Autodesk Inventor part; units mm, degrees
ref_plane "YZ Plane" through (0, 0, 0) normal (1, 0, 0) x (0, 1, 0)
ref_plane "XZ Plane" through (0, 0, 0) normal (0, 1, 0) x (-1, 0, 0)
ref_plane "XY Plane" through (0, 0, 0) normal (0, 0, 1) x (1, 0, 0)
sketch "Sketch1" plane through (0, 0, 0) normal (0, 0, 1) x (1, 0, 0)
  line L0 (0, 0) -> (15, 0)
  line L1 (15, 0) -> (15, 10)
  line L2 (15, 10) -> (0, 10)
  line L3 (0, 10) -> (0, 0)
  line L4 (1, 9) -> (14, 9)
  line L5 (14, 9) -> (14, 1)
  line L6 (14, 1) -> (1, 1)
  line L7 (1, 1) -> (1, 9)
  dimension "d0" = 15
  dimension "d1" = 10
  dimension "d2" = 13
  dimension "d3" = 8
  dimension "d4" = 1
  dimension "d5" = 1
extrude "Extrusion1" add sketch "Sketch1" along normal blind 28
sketch "Sketch2" plane through (0, 10, 0) normal (0, 1, 0) x (1, 0, 0)
  line L0 (15, 0) -> (0, 0)
  line L1 (0, 0) -> (0, -28)
  line L2 (15, -28) -> (0, -28)
  line L3 (15, 0) -> (15, -28)
  circle A0 centre (7.5, -5) radius 1.5
  circle A1 centre (7.5, -18) radius 1.5
  dimension "d8" = 3
  dimension "d9" = 3
  dimension "d10" = 7.5
  dimension "d11" = 7.5
  dimension "d12" = 5
  dimension "d13" = 10
extrude "Extrusion2" cut sketch "Sketch2" against normal up to surface (10 mm away) contours A0 | A1
sketch "Sketch3" plane through (15, 0, 0) normal (1, 0, 0) x (0, 0, -1)
  line L0 (0, 0) -> (0, 10)
  line L1 (0, 10) -> (-28, 10)
  line L2 (-28, 0) -> (-28, 10)
  line L3 (0, 0) -> (-28, 0)
  circle A0 centre (-9, 5) radius 1.5
  circle A1 centre (-23, 5) radius 1.5
  dimension "d16" = 3
  dimension "d17" = 5
  dimension "d18" = 9
  dimension "d21" = 3
  dimension "d22" = 5
  dimension "d23" = 5
extrude "Extrusion3" cut sketch "Sketch3" against normal up to surface (15 mm away) contours A0 | A1
properties part number "profile3" material "Aluminum 6061, Welded"
Source: CAD feature listing. Evaluate the final solid. Frame: model axes, mm. A direction names the side the tool comes from. Round coordinates to 2 decimals unless told otherwise and drop trailing zeros. Order: outer loops, then holes, each group sorted by start corner. A loop starts at its lowest first (then second) coordinate and runs counter-clockwise, first axis right, second up. Notation, with made-up numbers: (49, 60.5) -> (68, 60.5) arc R21 ccw to (68, 76.5) -> close; hole circle Ø6 at (51.25, -23.5). An arc over 180 degrees is marked (long way). Answer as CSV lines item,"result".
Item 1: Section B-B, the plane x = 7.5. Return loops of the section in (y, z).
A:
outline,"(0, 0) -> (1, 0) -> (1, 3.5) -> (0, 3.5) -> close; (0, 6.5) -> (1, 6.5) -> (1, 16.5) -> (0, 16.5) -> close; (0, 19.5) -> (1, 19.5) -> (1, 28) -> (0, 28) -> close; (9, 0) -> (10, 0) -> (10, 3.5) -> (9, 3.5) -> close; (9, 6.5) -> (10, 6.5) -> (10, 16.5) -> (9, 16.5) -> close; (9, 19.5) -> (10, 19.5) -> (10, 28) -> (9, 28) -> close"
Item 2: Section A-A, the plane y = 1.75. Return loops of the section in (x, z), plus the area to 3 significant figures.
A:
outline,"(0, 0) -> (1, 0) -> (1, 28) -> (0, 28) -> close; (14, 0) -> (15, 0) -> (15, 28) -> (14, 28) -> close"
area,"56.0 mm²"
Item 3: Section C-C, the plane z = 5. Return loops of the section in (x, y), plus the area to 3 significant figures.
A:
outline,"(0, 0) -> (6, 0) -> (6, 1) -> (1, 1) -> (1, 9) -> (6, 9) -> (6, 10) -> (0, 10) -> close; (9, 0) -> (15, 0) -> (15, 10) -> (9, 10) -> (9, 9) -> (14, 9) -> (14, 1) -> (9, 1) -> close"
area,"40.0 mm²"
Item 4: Line query: L1, parallel to Z at x = 7.5, y = 9.4; L2, parallel to Y at x = 13, z = 2.5; L3, parallel to Y at x = 0.7, z = 23. Output: solid intervals per line, ascending.
A:
L1,"0 to 3.5, 6.5 to 16.5, 19.5 to 28"
L2,"0 to 1, 9 to 10"
L3,"0 to 3.5, 6.5 to 10"
Item 5: Section D-D, the plane x = 10. Return loops of the section in (y, z), plus the area to 3 significant figures.
A:
outline,"(0, 0) -> (1, 0) -> (1, 28) -> (0, 28) -> close; (9, 0) -> (10, 0) -> (10, 28) -> (9, 28) -> close"
area,"56.0 mm²"
Item 6: Reachability of faces 4 (the face through (7, 0, 14)), 5 (the face through (1, 5, 14)) from +Z, -Z, +X, -X, +Y, -Y: full face, straight path, thin tool, end or side. Return the list, or none.
A:
face 4,"+Z, -Z, +X, -X, -Y"
face 5,"+Z, -Z"
Item 7: Pull-direction query (Z, two-part tool) for faces 1 (the face through (6.39, 9.51, 3.99)), 2 (the face through (7.4, 0.6, 28)), 3 (the face through (8, 10, 14)); classes: pulls with the +Z half, pulls with the -Z half, needs draft (parallel to the pull), parting line crosses it, or undercut.
A:
face 1,"undercut"
face 2,"pulls with the +Z half"
face 3,"needs draft"
